from build123d import *

# Parameters (mm, degrees)
ESQUISSE1_R        = 1.925
BOSS_EXTRU_1_DEPTH = 5


with BuildPart() as part:
    # Esquisse1 → Boss.-Extru.1 (new body)
    with BuildSketch(Plane.XY):
        with BuildLine():
            ThreePointArc((-55.827782292, -14.46282996), (24.922748014, -14.598984118), (105.525948354, -9.721405027))
            ThreePointArc((105.525948354, -9.721405027), (113.679539111, -0.101767596), (104.211594017, 8.227487007))
            ThreePointArc((104.211594017, 8.227487007), (30.47680307, 7.057280789), (-43.126605449, 11.609975917))
            ThreePointArc((-43.126605449, 11.609975917), (-46.576807991, 12.376745737), (-49.75182207, 13.929523614))
            ThreePointArc((-49.75182207, 13.929523614), (-54.116731069, 15.47051298), (-58.707950184, 14.880779279))
            ThreePointArc((-58.707950184, 14.880779279), (-82.908915105, 10.07391595), (-107.360082719, 13.380430803))
            ThreePointArc((-107.360082719, 13.380430803), (-114.932002243, 9.181129893), (-110.424129779, 1.788756847))
            ThreePointArc((-110.424129779, 1.788756847), (-86.236289716, -4.6172752), (-62.66641753, -13.016678668))
            ThreePointArc((-62.66641753, -13.016678668), (-59.310767285, -14.040827891), (-55.827782292, -14.46282996))
        make_face()
        with Locations((-23.472610973, -2.725250912)):
            Circle(ESQUISSE1_R, mode=Mode.SUBTRACT)
        with Locations((79.612874717, -2.574784989)):
            Circle(ESQUISSE1_R, mode=Mode.SUBTRACT)
        with Locations((-109.131234319, 7.647802958)):
            Circle(ESQUISSE1_R, mode=Mode.SUBTRACT)
        with Locations((-55.172918512, 5.526446001)):
            Circle(ESQUISSE1_R, mode=Mode.SUBTRACT)
        with Locations((104.703572766, -0.759056094)):
            Circle(ESQUISSE1_R, mode=Mode.SUBTRACT)
    extrude(amount=BOSS_EXTRU_1_DEPTH)


solid = part.part
Can you work these out from the model? Positions are in its coordinate system, mm. Round coordinates to 2 decimals unless told otherwise and drop trailing zeros. Loops run counter-clockwise (first coordinate to the right, second up) from the corner with the lowest first, then second, coordinate; pieces in that order, holes last. Notation, with made-up numbers: (75.5, 0) - (123.5, 0) arc R6 cw to (123.5, 8) - close; hole circle Ø1 at (88.25, 56.5). An arc over 180 degrees is marked (long way). Write item = value, one per line. Start each with the question number.
(1) If we section it at B-B (x = 88): Please give me the cut outline in (y, z), and give its area (3 significant figures).
(2) If we section it at C-C (x = -17): Please give me the cut outline in (y, z), and give its area (3 significant figures).
(3) For P1, Ø3, axis at x = -109.13, y = 7.65, coming from the -Z side; P2, Ø2, axis at x = 8.5, z = 4, coming from the -Y side, each with a flat end and sliding along its axis, tell me the tip position at first contact or that it passes through.
(4) If I drill on probe 1 along X at (y, z) = (6.5, 1.45); probe 2 along X at (y, z) = (6, 3.9); probe 3 along Y at (x, z) = (-54, 1.85), over which ranges is the centre line in solid material (lowest first)? Write a range as [from, to].
(5) If we mould it in two halves opening along Y, with no side actions, what happens to faces 1 (the face through (23.79, -14.63, 2.46)), 2 (the face through (-53.337, 6.105, 2.465)), 3 (the face through (31.509, 7.034, 2.465))? For each: released by +Y, released by -Y, zero draft, split by the parting line, or undercut.
(6) If we section it at A-A (z = 3): Give the number of separate pieces and of enclosed holes in the cut face, and give its area (3 significant figures).
Ans:
q1.outline = (-11.21, 0) - (7.48, 0) - (7.48, 5) - (-11.21, 5) - close
q1.area = 93.4 mm²
q2.outline = (-15.15, 0) - (9.34, 0) - (9.34, 5) - (-15.15, 5) - close
q2.area = 122 mm²
q3.P1 = through
q3.P2 = -14.99
q4.probe_1 = [-115.02, -110.68], [-107.59, -56.83], [-53.51, 110.02]
q4.probe_2 = [-114.9, -110.13], [-108.14, -57.04], [-53.31, 110.65]
q4.probe_3 = [-14.52, 4], [7.05, 15.46]
q5.face_1 = released by -Y
q5.face_2 = undercut
q5.face_3 = released by +Y
q6.separate_pieces = 1
q6.enclosed_holes = 5
q6.area = 4,650 mm²
